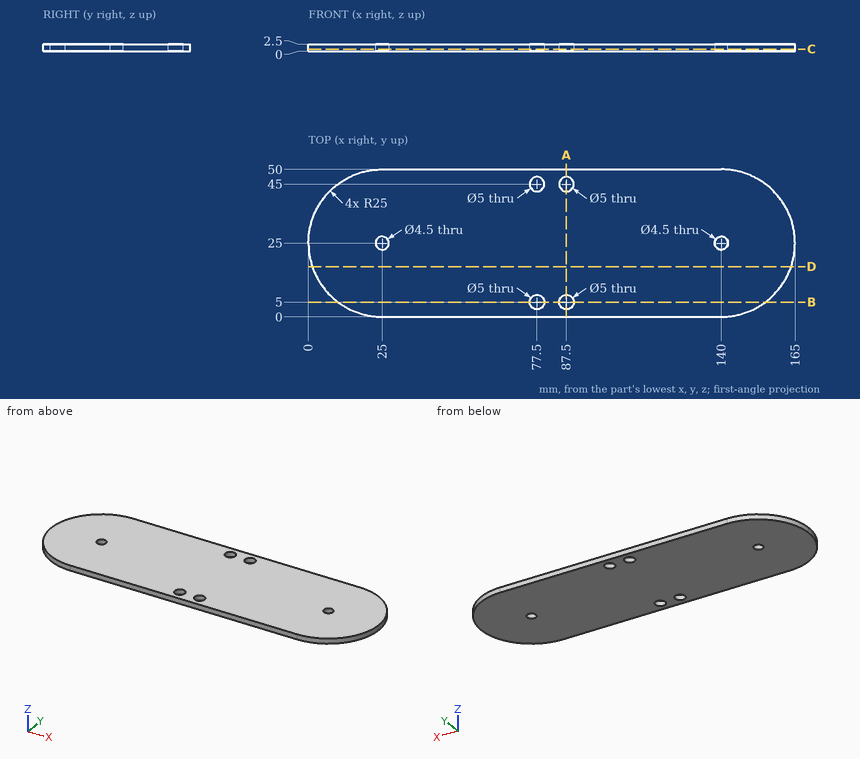
Answer from the drawing. Dimensions are ordinates in mm from the lowest x, y and z of the part. Give positions to 0.01 mm unless a question says otherwise; leave off trailing zeros. Order: outer loops, then holes, each group sorted by start corner. A loop starts at its lowest first (then second) coordinate and runs counter-clockwise, first axis right, second up. Notation, with made-up numbers: (29.5, -17) -> (67.5, -17) arc R11 ccw to (67.5, -4) -> close; hole circle Ø1 at (-30.5, 87.25). An arc over 180 degrees is marked (long way). Answer as a JSON object with one key per item and string values. Group by question number.
1. Consider line 1 along Y through (x, z) = (77.5, 1.95); line 2 along Y through (x, z) = (89, 1.1); line 3 along X through (y, z) = (43, 0.4). Determine where each line is inside the solid, lowest interval first. Write a range as [from, to].
2. Section B-B on y = 5 is taken. Determine the outline of the cut face in (x, z).
3. Section D-D on y = 17 is taken. Determine the outline of the cut face in (x, z).
4. A flat-ended cylindrical pin translates along its axis: pin 1 Ø4 at (x, y) = (77.5, 5) entering from -Z. Find the tip coordinate at first contact, or state that the pin passes through.
5. Section A-A on x = 87.5 is taken. Determine the outline of the cut face in (y, z), plus the area to 3 significant figures.
6. Section C-C on z = 0.8 is taken. Count the separate pieces of the cut face and the enclosed holes in it, plus the area to 3 significant figures.
Result sheet:
{
 "1": {"line 1": "y = [0, 2.5], [7.5, 42.5], [47.5, 50]", "line 2": "y = [0, 3], [7, 43], [47, 50]", "line 3": "x = [7.65, 76], [79, 86], [89, 157.35]"},
 "2": {"outline": "(10, 0) -> (75, 0) -> (75, 2.5) -> (10, 2.5) -> close; (80, 0) -> (85, 0) -> (85, 2.5) -> (80, 2.5) -> close; (90, 0) -> (155, 0) -> (155, 2.5) -> (90, 2.5) -> close"},
 "3": {"outline": "(1.31, 0) -> (163.69, 0) -> (163.69, 2.5) -> (1.31, 2.5) -> close"},
 "4": {"pin 1": "passes through"},
 "5": {"outline": "(0, 0) -> (2.5, 0) -> (2.5, 2.5) -> (0, 2.5) -> close; (7.5, 0) -> (42.5, 0) -> (42.5, 2.5) -> (7.5, 2.5) -> close; (47.5, 0) -> (50, 0) -> (50, 2.5) -> (47.5, 2.5) -> close", "area": "100 mm^2"},
 "6": {"separate pieces": "1", "enclosed holes": "6", "area": "7,600 mm^2"}
}
